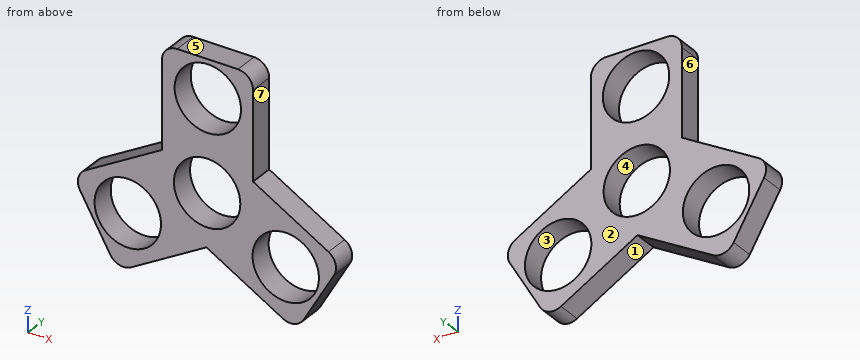
from build123d import *

# Parameters (mm, degrees)
F0_R     = 10.925
F1_DEPTH = 8


with BuildPart() as f1:
    # F0 (on Front) → F1 (new body)
    with BuildSketch(Plane.XZ):
        with BuildLine():
            Line((-136.3183801476, -4.150791151), (-136.3183801476, -8.1894561753))
            Line((-136.3183801476, -8.1894561753), (-143.3135531644, -8.1894561753))
            Line((-143.3135531644, -8.1894561753), (-151.6621599046, -13.0095265241))
            Line((-151.6621599046, -13.0095265241), (-126.5146964668, -27.5284213094))
            ThreePointArc((-126.5146964668, -27.5284213094), (-122.7206012413, -28.027923422), (-119.6845694479, -25.6982942905))
            Line((-119.6845694479, -25.6982942905), (-109.6845694479, -8.3777862148))
            ThreePointArc((-109.6845694479, -8.3777862148), (-109.1850673353, -4.5836909893), (-111.5146964668, -1.5476591959))
            Line((-111.5146964668, -1.5476591959), (-136.3183801476, 12.7727542541))
            Line((-136.3183801476, 12.7727542541), (-136.3183801476, 3.1326135564))
            Line((-136.3183801476, 3.1326135564), (-133.1645733963, -2.3299399742))
            Line((-133.1645733963, -2.3299399742), (-136.3183801476, -4.150791151))
        make_face()
        with Locations((-125.5675627039, -10.8870620569)):
            Circle(F0_R, mode=Mode.SUBTRACT)
        Polygon((-144.6669868879, 17.592824603), (-136.3183801476, 3.1326135564), (-136.3183801476, 12.7727542541), align=None)
        Polygon((-157.9697734074, 17.9897872735), (-151.6621599046, 21.6314896272), (-154.815966656, 23.4523408041), align=None)
        with BuildLine():
            Line((-144.6669868879, 17.592824603), (-136.3183801476, 12.7727542541))
            Line((-136.3183801476, 12.7727542541), (-136.3183801476, 41.8105438247))
            ThreePointArc((-136.3183801476, 41.8105438247), (-137.7828462417, 45.3460777306), (-141.3183801476, 46.8105438247))
            Line((-141.3183801476, 46.8105438247), (-161.3183801476, 46.8105438247))
            ThreePointArc((-161.3183801476, 46.8105438247), (-164.8539140536, 45.3460777306), (-166.3183801476, 41.8105438247))
            Line((-166.3183801476, 41.8105438247), (-166.3183801476, 13.1697169246))
            Line((-166.3183801476, 13.1697169246), (-157.9697734074, 17.9897872735))
            Line((-157.9697734074, 17.9897872735), (-154.815966656, 23.4523408041))
            Line((-154.815966656, 23.4523408041), (-151.6621599046, 21.6314896272))
            Line((-151.6621599046, 21.6314896272), (-148.1645733963, 23.6508221394))
            Line((-148.1645733963, 23.6508221394), (-144.6669868879, 17.592824603))
        make_face()
        with Locations((-151.2037868953, 34.3101060979)):
            Circle(F0_R, mode=Mode.SUBTRACT)
        Polygon((-166.3183801476, 13.1697169246), (-166.3183801476, 3.5295762269), (-157.9697734074, 17.9897872735), align=None)
        with BuildLine():
            Line((-151.6621599046, -13.0095265241), (-160.0107666449, -8.1894561753))
            Line((-160.0107666449, -8.1894561753), (-166.3183801476, -8.1894561753))
            Line((-166.3183801476, -8.1894561753), (-166.3183801476, -4.5477538216))
            Line((-166.3183801476, -4.5477538216), (-169.815966656, -2.5284213094))
            Line((-169.815966656, -2.5284213094), (-166.3183801476, 3.5295762269))
            Line((-166.3183801476, 3.5295762269), (-166.3183801476, 13.1697169246))
            Line((-166.3183801476, 13.1697169246), (-191.4658435855, -1.3491778606))
            ThreePointArc((-191.4658435855, -1.3491778606), (-193.7954727169, -4.3852096541), (-193.2959706044, -8.1793048796))
            Line((-193.2959706044, -8.1793048796), (-183.2959706044, -25.4998129553))
            ThreePointArc((-183.2959706044, -25.4998129553), (-180.259938811, -27.8294420867), (-176.4658435855, -27.3299399742))
            Line((-176.4658435855, -27.3299399742), (-151.6621599046, -13.0095265241))
        make_face()
        with Locations((-177.5275706007, -10.4900993864)):
            Circle(F0_R, mode=Mode.SUBTRACT)
        Polygon((-160.0107666449, -8.1894561753), (-143.3135531644, -8.1894561753), (-136.3183801476, -4.150791151), (-136.3183801476, 3.1326135564), (-144.6669868879, 17.592824603), (-151.6621599046, 21.6314896272), (-157.9697734074, 17.9897872735), (-166.3183801476, 3.5295762269), (-166.3183801476, -4.5477538216), align=None)
        with Locations((-151.4329734, 4.3109815515)):
            Circle(F0_R, mode=Mode.SUBTRACT)
        Polygon((-169.815966656, -2.5284213094), (-166.3183801476, -4.5477538216), (-166.3183801476, 3.5295762269), align=None)
        Polygon((-151.6621599046, 21.6314896272), (-144.6669868879, 17.592824603), (-148.1645733963, 23.6508221394), align=None)
        Polygon((-136.3183801476, 3.1326135564), (-136.3183801476, -4.150791151), (-133.1645733963, -2.3299399742), align=None)
        Polygon((-143.3135531644, -8.1894561753), (-136.3183801476, -8.1894561753), (-136.3183801476, -4.150791151), align=None)
        Polygon((-166.3183801476, -8.1894561753), (-160.0107666449, -8.1894561753), (-166.3183801476, -4.5477538216), align=None)
        Polygon((-151.6621599046, -13.0095265241), (-143.3135531644, -8.1894561753), (-160.0107666449, -8.1894561753), align=None)
    extrude(amount=F1_DEPTH)


solid = f1.part
The model under review builds one solid part; all positions refer to its coordinate system, in mm. Face numbers are marked on the shaded views. A direction names the side the tool comes from. Round coordinates to 2 decimals unless told otherwise and drop trailing zeros. Order: outer loops, then holes, each group sorted by start corner. A loop starts at its lowest first (then second) coordinate and runs counter-clockwise, first axis right, second up. Notation, with made-up numbers: (-36, -16) -> (-31, -16) arc R22 ccw to (-31, 7) -> close; hole circle Ø7 at (-25.75, -19.75). An arc over 180 degrees is marked (long way). Write item = value, one per line. Start each with the question number.
Item 1: Clearance check with flat-ended pins moving along their axes: pin 1 Ø25 at (x, z) = (-177.53, -10.49) entering from +Y; pin 2 Ø3 at (x, y) = (-135, -1.5) entering from -Z; pin 3 Ø3 at (x, y) = (-174.5, -5) entering from -Z; pin 4 Ø2 at (x, y) = (-148, -6) entering from -Z. State where each tip first meets the part, or that it passes through.
Item 2: Mouldability with a two-part tool opening along Z and no side actions: class the marked faces 1, 2, 3 and 4 as released by +Z, released by -Z, zero draft, split by the parting line, or undercut.
Item 3: For the marked faces 5, 6 and 7, list the 3-axis set-ups (+Z, -Z, +X, -X, +Y, -Y) from which the entire face can be reached by the end or side of a thin tool; tool diameter is ignored.
Item 4: Consider section B-B on x = -173.5. Write out the cut boundary in (y, z), plus the area to 3 significant figures.
Item 5: Consider section C-C on y = -2. Write out the cut boundary in (x, z) (3 decimals), plus the area to 3 significant figures.
Item 6: Consider section A-A on z = 1.5. Write out the cut boundary in (x, y).
Item 7: For line 1 along X through (y, z) = (-0.5, -12); line 2 along X through (y, z) = (-3, -15.5); line 3 along Z through (x, y) = (-150.5, -4.75), list the stretches that pass through material, from the lowest coordinate up.
Conclusion:
q1.pin_1 = 0
q1.pin_2 = -23.5
q1.pin_3 = -27.06
q1.pin_4 = -15.7
q2.face_1 = released by -Z
q2.face_2 = zero draft
q2.face_3 = undercut
q2.face_4 = undercut
q3.face_5 = +Z, +X, -X, +Y, -Y
q3.face_6 = +Z, -X, +Y, -Y
q3.face_7 = +Z, +X, +Y, -Y
q4.outline = (-8, -25.62) -> (0, -25.62) -> (0, -20.65) -> (-8, -20.65) -> close; (-8, -0.33) -> (0, -0.33) -> (0, 9.02) -> (-8, 9.02) -> close
q4.area = 115 mm2
q5.outline = (-193.296, -8.179) -> (-183.296, -25.5) arc R5 ccw to (-176.466, -27.33) -> (-151.662, -13.01) -> (-126.515, -27.528) arc R5 ccw to (-119.685, -25.698) -> (-109.685, -8.378) arc R5 ccw to (-111.515, -1.548) -> (-136.318, 12.773) -> (-136.318, 41.811) arc R5 ccw to (-141.318, 46.811) -> (-161.318, 46.811) arc R5 ccw to (-166.318, 41.811) -> (-166.318, 13.17) -> (-191.466, -1.349) arc R5 ccw to start; hole circle Ø21.85 at (-177.528, -10.49); hole circle Ø21.85 at (-151.433, 4.311); hole circle Ø21.85 at (-151.204, 34.31); hole circle Ø21.85 at (-125.568, -10.887)
q5.area = 1,900 mm2
q6.outline = (-186.53, -8) -> (-161.99, -8) -> (-161.99, 0) -> (-186.53, 0) -> close; (-140.88, -8) -> (-116.79, -8) -> (-116.79, 0) -> (-140.88, 0) -> close
q7.line_1 = -191.09 to -188.35, -166.71 to -136.44, -114.7 to -111.78
q7.line_2 = -189.07 to -187.24, -167.82 to -155.98, -147.35 to -135.47, -115.66 to -113.8
q7.line_3 = -13.68 to -6.57, 15.2 to 23.41, 45.21 to 46.81
